from build123d import *

# Parameters (mm, degrees)
SKETCH_1_W          = 17.09
SKETCH_1_H          = 28.3
EXTRUDE_1_DEPTH     = 25.25
EXTRUDE_2_DEPTH     = 0.3
EXTRUDE_START       = -0.3
EXTRUDE_3_DEPTH     = 0.3
EXTRUDE_4_DEPTH     = 3.3
SKETCH_7_R          = 0.25
EXTRUDE_5_DEPTH     = 3.15
FILLET_1_R          = 0.3
CUT_EXTRUDE_1_DEPTH = 10
EXTRUDE_6_DEPTH     = 9.7
SKETCH_10_W         = 2.6
SKETCH_10_H         = 1.5
EXTRUDE_7_DEPTH     = 0.1
EXTRUDE_8_DEPTH     = 9.7


with BuildPart() as part:
    # 草图1 → 凸台-拉伸1 (new body)
    with BuildSketch(Plane(origin=(0, 0, 0), x_dir=(1, 0, 0), z_dir=(0, 1, 0))):
        with Locations((8.545, 14.15)):
            Rectangle(SKETCH_1_W, SKETCH_1_H)
    extrude(amount=EXTRUDE_1_DEPTH)

    # 草图2 → 凸台-拉伸2 (add)
    with BuildSketch(Plane(origin=(17.09, 0, 0), x_dir=(0, 0, -1), z_dir=(1, 0, 0))):
        with BuildLine():
            Line((21.62, 0), (21.62, -3.45))
            ThreePointArc((21.62, -3.45), (22.27, -4.1), (22.92, -3.45))
            Line((22.92, -3.45), (22.92, 0))
            Line((22.92, 0), (21.62, 0))
        make_face()
        with BuildLine():
            Line((6.92, -3.45), (6.92, 0))
            Line((6.92, 0), (5.62, 0))
            Line((5.62, 0), (5.62, -3.45))
            ThreePointArc((5.62, -3.45), (6.27, -4.1), (6.92, -3.45))
        make_face()
    extrude(amount=-EXTRUDE_2_DEPTH)

    # 草图4 → 凸台-拉伸3 (add)
    with BuildSketch(Plane.ZY.offset(EXTRUDE_START)):
        with BuildLine():
            Line((-5.62, -3.45), (-5.62, 0))
            Line((-5.62, 0), (-6.92, 0))
            Line((-6.92, 0), (-6.92, -3.45))
            ThreePointArc((-6.92, -3.45), (-6.27, -4.1), (-5.62, -3.45))
        make_face()
        with BuildLine():
            Line((-25.68, -3.45), (-25.68, 0))
            Line((-25.68, 0), (-26.98, 0))
            Line((-26.98, 0), (-26.98, -3.45))
            ThreePointArc((-26.98, -3.45), (-26.33, -4.1), (-25.68, -3.45))
        make_face()
    extrude(amount=EXTRUDE_3_DEPTH)

    # 草图5 → 凸台-拉伸4 (add)
    with BuildSketch(Plane.XZ):
        with BuildLine():
            ThreePointArc((1.306965866, -10.552133668), (1.28, -10.84), (1.306965866, -11.127866332))
            ThreePointArc((1.306965866, -11.127866332), (2.122893219, -11.547106781), (2.542133668, -12.363034134))
            ThreePointArc((2.542133668, -12.363034134), (2.83, -12.39), (3.117866332, -12.363034134))
            ThreePointArc((3.117866332, -12.363034134), (3.537106781, -11.547106781), (4.353034134, -11.127866332))
            ThreePointArc((4.353034134, -11.127866332), (4.38, -10.84), (4.353034134, -10.552133668))
            ThreePointArc((4.353034134, -10.552133668), (3.537106781, -10.132893219), (3.117866332, -9.316965866))
            ThreePointArc((3.117866332, -9.316965866), (2.83, -9.29), (2.542133668, -9.316965866))
            ThreePointArc((2.542133668, -9.316965866), (2.122893219, -10.132893219), (1.306965866, -10.552133668))
        make_face()
        with BuildLine():
            ThreePointArc((14.547866332, -12.363034134), (14.26, -12.39), (13.972133668, -12.363034134))
            ThreePointArc((13.972133668, -12.363034134), (13.552893219, -11.547106781), (12.736965866, -11.127866332))
            ThreePointArc((12.736965866, -11.127866332), (12.71, -10.84), (12.736965866, -10.552133668))
            ThreePointArc((12.736965866, -10.552133668), (13.552893219, -10.132893219), (13.972133668, -9.316965866))
            ThreePointArc((13.972133668, -9.316965866), (14.26, -9.29), (14.547866332, -9.316965866))
            ThreePointArc((14.547866332, -9.316965866), (14.967106781, -10.132893219), (15.783034134, -10.552133668))
            ThreePointArc((15.783034134, -10.552133668), (15.81, -10.84), (15.783034134, -11.127866332))
            ThreePointArc((15.783034134, -11.127866332), (14.967106781, -11.547106781), (14.547866332, -12.363034134))
        make_face()
    extrude(amount=EXTRUDE_4_DEPTH)

    # 草图7 → 凸台-拉伸5 (add)
    with BuildSketch(Plane.XZ):
        with Locations(Location((5.5, -13.65, 0), (0, 0, 90))):
            Circle(SKETCH_7_R)
        with Locations(Location((7.53, -13.65, 0), (0, 0, 90))):
            Circle(SKETCH_7_R)
        with Locations(Location((5.5, -11.85, 0), (0, 0, 90))):
            Circle(SKETCH_7_R)
        with Locations(Location((7.53, -11.85, 0), (0, 0, 90))):
            Circle(SKETCH_7_R)
        with Locations(Location((9.56, -11.85, 0), (0, 0, 90))):
            Circle(SKETCH_7_R)
        with Locations(Location((11.59, -11.85, 0), (0, 0, 90))):
            Circle(SKETCH_7_R)
        with Locations(Location((9.56, -13.65, 0), (0, 0, 90))):
            Circle(SKETCH_7_R)
        with Locations(Location((11.59, -13.65, 0), (0, 0, 90))):
            Circle(SKETCH_7_R)
        with Locations(Location((5.245, -15.54, 0), (0, 0, 90))):
            Circle(SKETCH_7_R)
        with Locations(Location((6.515, -16.81, 0), (0, 0, 90))):
            Circle(SKETCH_7_R)
        with Locations(Location((5.245, -18.077907843, 0), (0, 0, 90))):
            Circle(SKETCH_7_R)
        with Locations(Location((6.515, -19.347907843, 0), (0, 0, 90))):
            Circle(SKETCH_7_R)
        with Locations(Location((5.245, -20.615815685, 0), (0, 0, 90))):
            Circle(SKETCH_7_R)
        with Locations(Location((6.515, -21.885815685, 0), (0, 0, 90))):
            Circle(SKETCH_7_R)
        with Locations(Location((6.515, -24.423723528, 0), (0, 0, 90))):
            Circle(SKETCH_7_R)
        with Locations(Location((5.245, -25.69163137, 0), (0, 0, 90))):
            Circle(SKETCH_7_R)
        with Locations(Location((5.245, -23.153723528, 0), (0, 0, 90))):
            Circle(SKETCH_7_R)
        with Locations(Location((6.515, -26.96163137, 0), (0, 0, 90))):
            Circle(SKETCH_7_R)
        with Locations(Location((10.575, -26.96163137, 0), (0, 0, 90))):
            Circle(SKETCH_7_R)
        with Locations(Location((11.845, -23.153723528, 0), (0, 0, 90))):
            Circle(SKETCH_7_R)
        with Locations(Location((11.845, -25.69163137, 0), (0, 0, 90))):
            Circle(SKETCH_7_R)
        with Locations(Location((10.575, -24.423723528, 0), (0, 0, 90))):
            Circle(SKETCH_7_R)
        with Locations(Location((10.575, -21.885815685, 0), (0, 0, 90))):
            Circle(SKETCH_7_R)
        with Locations(Location((11.845, -20.615815685, 0), (0, 0, 90))):
            Circle(SKETCH_7_R)
        with Locations(Location((10.575, -19.347907843, 0), (0, 0, 90))):
            Circle(SKETCH_7_R)
        with Locations(Location((11.845, -18.077907843, 0), (0, 0, 90))):
            Circle(SKETCH_7_R)
        with Locations(Location((10.575, -16.81, 0), (0, 0, 90))):
            Circle(SKETCH_7_R)
        with Locations(Location((11.845, -15.54, 0), (0, 0, 90))):
            Circle(SKETCH_7_R)
    extrude(amount=EXTRUDE_5_DEPTH)

    # 圆角1
    fillet_1_edges = [part.edges().sort_by_distance(p)[0] for p in [
        (17.09, 25.25, -14.15),
        (8.545, 25.25, -28.3),
        (0, 25.25, -14.15),
        (8.545, 0, 0),
        (0, 12.625, -28.3),
        (17.09, 12.625, -28.3),
        (17.09, 12.625, 0),
        (0, 12.625, 0),
        (8.545, 25.25, 0),
    ]]
    fillet(fillet_1_edges, radius=FILLET_1_R)

    # 草图8 → 切除-拉伸1 (cut)
    with BuildSketch(Plane.XY):
        Polygon((15.045, 14.25), (2.045, 14.25), (2.045, 24.25), (6.145, 24.25), (6.145, 24.95), (10.945, 24.95), (10.945, 24.25), (15.045, 24.25), align=None)
        Polygon((10.945, 0.3), (6.145, 0.3), (6.145, 1), (2.045, 1), (2.045, 11), (15.045, 11), (15.045, 1), (10.945, 1), align=None)
    extrude(amount=-CUT_EXTRUDE_1_DEPTH, mode=Mode.SUBTRACT)

    # 草图9 → 凸台-拉伸6 (add)
    with BuildSketch(Plane.XY.offset(-10)):
        Polygon((2.045, 24.25), (2.045, 21.75), (5.045, 21.75), (5.045, 23.45), (6.345, 23.45), (6.345, 24.85), (10.745, 24.85), (10.745, 23.45), (12.045, 23.45), (12.045, 21.75), (15.045, 21.75), (15.045, 24.25), (10.945, 24.25), (10.945, 24.95), (6.145, 24.95), (6.145, 24.25), align=None)
        Polygon((15.045, 1), (15.045, 3.5), (12.045, 3.5), (12.045, 1.8), (10.745, 1.8), (10.745, 0.4), (6.345, 0.4), (6.345, 1.8), (5.045, 1.8), (5.045, 3.5), (2.045, 3.5), (2.045, 1), (6.145, 1), (6.145, 0.3), (10.945, 0.3), (10.945, 1), align=None)
    extrude(amount=EXTRUDE_6_DEPTH)

    # 草图10 → 凸台-拉伸7 (add)
    with BuildSketch(Plane.XY.offset(-0.3)):
        with Locations((3.345, 23.5)):
            Rectangle(SKETCH_10_W, SKETCH_10_H)
        with Locations((13.745, 23.5)):
            Rectangle(SKETCH_10_W, SKETCH_10_H)
        with Locations((13.745, 1.75)):
            Rectangle(SKETCH_10_W, SKETCH_10_H)
        with Locations((3.345, 1.75)):
            Rectangle(SKETCH_10_W, SKETCH_10_H)
    extrude(amount=EXTRUDE_7_DEPTH)

    # 草图11 → 凸台-拉伸8 (add)
    with BuildSketch(Plane.XY.offset(-10)):
        Polygon((15.045, 3.5), (15.045, 11), (2.045, 11), (2.045, 3.5), (2.345, 3.5), (2.345, 10.7), (14.745, 10.7), (14.745, 3.5), align=None)
        Polygon((14.745, 21.75), (15.045, 21.75), (15.045, 14.25), (2.045, 14.25), (2.045, 21.75), (2.345, 21.75), (2.345, 14.55), (14.745, 14.55), align=None)
    extrude(amount=EXTRUDE_8_DEPTH)


solid = part.part
Can you work these out from the model? Positions are in its coordinate system, mm. A direction names the side the tool comes from. Coordinates: 2 decimals unless noted, no trailing zeros. Loops run counter-clockwise (first coordinate to the right, second up) from the corner with the lowest first, then second, coordinate; pieces in that order, holes last. Notation, with made-up numbers: (-33.5, 86) - (-22.5, 86) arc R10 ccw to (-22.5, 90) - close; hole circle Ø6 at (44.5, 12). An arc over 180 degrees is marked (long way). Answer as a JSON object with one key per item and string values. Group by question number.
Item 1: If we section it at B-B (y = 15.75): List the corners of the cut face in (x, z) for me (3 decimals).
Item 2: If we mould it in two halves opening along X, with no side actions, what happens to faces 1 (the face through (17.09, 13, -14)), 2 (the face through (4, 3.5, -5)), 3 (the face through (14, -3.3, -11))? For each: released by +X, released by -X, zero draft, split by the parting line, or undercut.
Item 3: If I drill on L1, parallel to Y at x = 11, z = -8; L2, parallel to X at y = 7, z = -2.75 (3 decimals); L3, parallel to Z at x = 3, y = 6.25, over which ranges is the centre line in solid material (lowest first)? Write a range as from..to.
Item 4: For pin 1 (2.5 mm diameter, centred on x = 3, z = -11, fed in from -Y); pin 2 (3 mm diameter, centred on x = 11.5, y = 19.5, fed in from +Z); pin 3 (2 mm diameter, centred on x = 13, z = -20, fed in from -Y); pin 4 (12 mm diameter, centred on y = 16, z = -22.5, fed in from -X), each with a flat end and sliding along its axis, tell me the tip position at first contact or that it passes through.
Item 5: If we section it at C-C (z = -13): List the corners of the cut face in (x, y) for me, plus the area to 3 significant figures.
Item 6: If we section it at A-A (z = -6.27): State how many separate pieces and enclosed holes the cut face has, plus the area to 3 significant figures.
Item 7: On a 3-axis mill with a long thin cutter (end or side, diameter ignored), from which of +Z, -Z, +X, -X, +Y, -Y can I reach the whole of each face in a straight line? I mean faces 4 (the face through (14, 2, -0.2)), 5 (the face through (16.79, -2, -22)), 6 (the face through (14.958, -1.627, -10.124)). Say none if no direction works.
Returned:
{
 "1": {"outline": "(0, -28) arc R0.3 ccw to (0.3, -28.3) - (16.79, -28.3) arc R0.3 ccw to (17.09, -28) - (17.09, -0.3) arc R0.3 ccw to (16.79, 0) - (15.045, 0) - (15.045, -0.3) - (14.745, -0.3) - (14.745, -10) - (2.345, -10) - (2.345, -0.3) - (2.045, -0.3) - (2.045, 0) - (0.3, 0) arc R0.3 ccw to (0, -0.3) - close"},
 "2": {"face 1": "released by +X", "face 2": "undercut", "face 3": "zero draft"},
 "3": {"L1": "y = 0..1.8, 10.7..14.55, 23.45..25.25", "L2": "x = 0..2.345, 14.745..17.09", "L3": "z = -28.3..-10"},
 "4": {"pin 1": "stops at y = -3.3", "pin 2": "stops at z = -10", "pin 3": "stops at y = 0", "pin 4": "stops at x = 0"},
 "5": {"outline": "(0, 0) - (17.09, 0) - (17.09, 24.95) arc R0.3 ccw to (16.79, 25.25) - (0.3, 25.25) arc R0.3 ccw to (0, 24.95) - close", "area": "431 mm²"},
 "6": {"separate pieces": "1", "enclosed holes": "2", "area": "219 mm²"},
 "7": {"face 4": "+Z", "face 5": "+Z, -Z, -Y", "face 6": "+Z, +X, -Y"}
}
